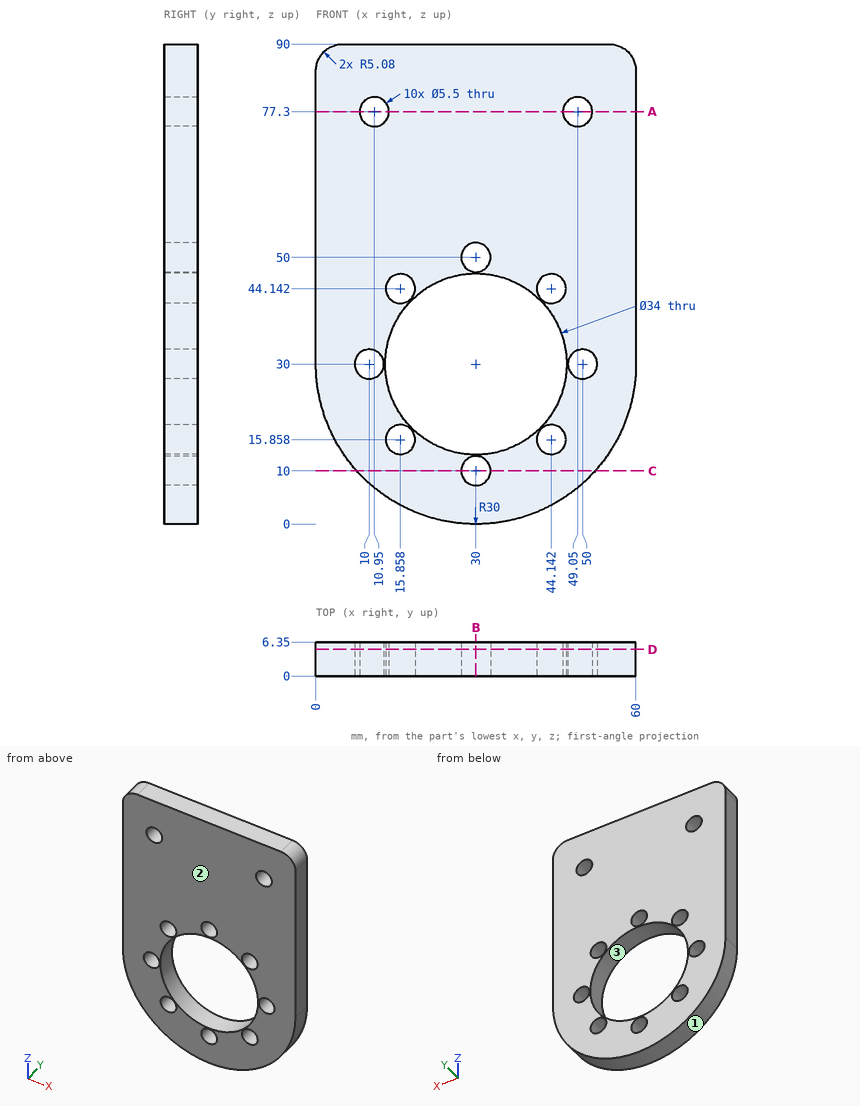
Part print with two shaded views. Sizes in mm from the minimum x, y, z corner. Round coordinates to 2 decimals unless told otherwise and drop trailing zeros. Write each loop counter-clockwise with the first axis right and the second up, starting at its lowest first coordinate (ties: lowest second). Pieces come first, ordered by that corner, then holes. Notation, with made-up numbers: (75.25, 64) - (95.25, 64) arc R29 cw to (95.25, 88) - close; hole circle Ø3 at (66.5, 41). An arc over 180 degrees is marked (long way). Answer as CSV lines item,"result".
Q1. Cut at A-A (z = 77.3). Write the cut outline in (x, y).
Report:
outline,"(0, 0) - (8.2, 0) - (8.2, 6.35) - (0, 6.35) - close; (13.7, 0) - (46.3, 0) - (46.3, 6.35) - (13.7, 6.35) - close; (51.8, 0) - (60, 0) - (60, 6.35) - (51.8, 6.35) - close"
Q2. Cut at C-C (z = 10). Write the cut outline in (x, y), and give its area (3 significant figures).
Report:
outline,"(7.64, 0) - (27.25, 0) - (27.25, 6.35) - (7.64, 6.35) - close; (32.75, 0) - (52.36, 0) - (52.36, 6.35) - (32.75, 6.35) - close"
area,"249 mm^2"
Q3. Pull direction X, two halves, no side cores. Call the marked faces 1, 2 and 3: +X half, -X half, draft (parallel to the pull), parting line (faces both ways), or undercut.
Report:
face 1,"parting line"
face 2,"draft"
face 3,"undercut"
Q4. Cut at B-B (x = 30). Write the cut outline in (y, z).
Report:
outline,"(0, 0) - (6.35, 0) - (6.35, 7.25) - (0, 7.25) - close; (0, 12.75) - (6.35, 12.75) - (6.35, 13) - (0, 13) - close; (0, 47) - (6.35, 47) - (6.35, 47.25) - (0, 47.25) - close; (0, 52.75) - (6.35, 52.75) - (6.35, 90) - (0, 90) - close"
Q5. Drop flat-ended pins along their axis: pin 1 (3.5 mm diameter, centred on x = 15.86, z = 15.86, fed in from +Y); pin 2 (10 mm diameter, centred on x = 40, z = 58.5, fed in from -Y); pin 3 (1.5 mm diameter, centred on x = 36.5, y = 5.5, fed in from -Z). Give the stop position or say it passes through.
Report:
pin 1,"passes through"
pin 2,"stops at y = 0"
pin 3,"stops at z = 0.56"
Q6. Drill centre lines: probe 1 along Z at (x, y) = (18, 3.75) (1 decimal); probe 2 along Z at (x, y) = (11, 6.25); probe 3 along Z at (x, y) = (51, 3) (1 decimal). Where is each one in solid material? Low to high. Write a range as [from, to].
Report:
probe 1,"z = [2.5, 14.1], [17.6, 18], [42, 42.4], [45.9, 90]"
probe 2,"z = [6.78, 27.44], [32.56, 74.55], [80.05, 90]"
probe 3,"z = [8.6, 27.4], [32.6, 75.4], [79.2, 90]"
Q7. Cut at D-D (y = 5). State how many separate pieces and enclosed holes the cut face has, and give its area (3 significant figures).
Report:
separate pieces,"1"
enclosed holes,"11"
area,"3,860 mm^2"
